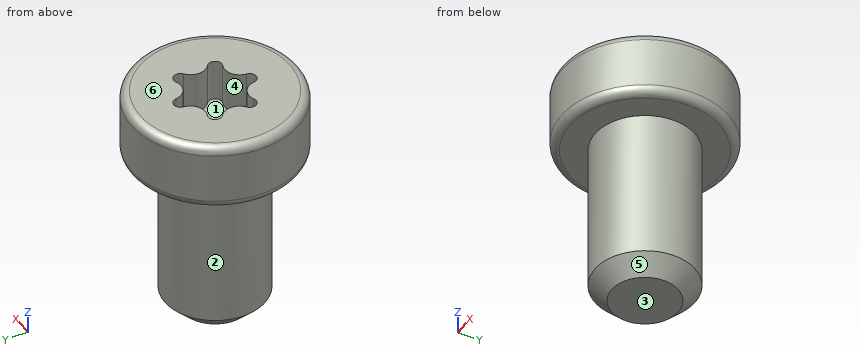
Solid Edge part; units mm, degrees
sketch "Sketch1" plane through (0, 0, 0) normal (0, -1, 0) x (1, 0, 0)
  line L0 (0, 4) -> (5, 4)
  line L1 (5, 4) -> (5, 0)
  line L2 (5, 0) -> (3, 0)
  line L3 (3, 0) -> (3, -10)
  line L4 (3, -10) -> (0, -10)
  line L5 (0, -10) -> (0, 4)
  dimension "D1" = 3
  dimension "D2" = 3
  dimension "D3" = 5
revolve "RevolvedProtrusion1" add sketch "Sketch1" angle 360 about axis through (0, 0, 54) along (0, 0, -1)
sketch "Sketch2" plane through (0, 0, 4) normal (0, 0, 1) x (1, 0, 0)
  arc A0 (-2.0545, -0.7268) -> (-1.6567, -1.4158) centre (-1.8186, -1.05) ccw
  arc A1 (-1.6567, -1.4158) -> (-0.3978, -2.1427) centre (-1.2926, -2.2389) cw
  arc A2 (-0.3978, -2.1427) -> (0.3978, -2.1427) centre (0, -2.0999) ccw
  arc A3 (0.3978, -2.1427) -> (1.6567, -1.4158) centre (1.2926, -2.2389) cw
  arc A4 (1.6567, -1.4158) -> (2.0545, -0.7268) centre (1.8186, -1.05) ccw
  arc A5 (2.0545, -0.7268) -> (2.0545, 0.7268) centre (2.5853, 0) cw
  arc A6 (2.0545, 0.7268) -> (1.6567, 1.4158) centre (1.8186, 1.05) ccw
  arc A7 (1.6567, 1.4158) -> (0.3978, 2.1427) centre (1.2926, 2.2389) cw
  arc A8 (0.3978, 2.1427) -> (-0.3978, 2.1427) centre (0, 2.0999) ccw
  arc A9 (-0.3978, 2.1427) -> (-1.6567, 1.4158) centre (-1.2926, 2.2389) cw
  arc A10 (-1.6567, 1.4158) -> (-2.0545, 0.7268) centre (-1.8186, 1.05) ccw
  arc A11 (-2.0545, 0.7268) -> (-2.0545, -0.7268) centre (-2.5853, 0) cw
extrude "Cutout1" cut sketch "Sketch2" against normal blind 2.5
fillet "Verrundung_1" radius 0.5 2 edges at (-5, 0, 4) (-5, 0, 0)
chamfer "Fase_1" distance 1 angle 45 1 edges at (-3, 0, -10)
The listing builds one solid part. Answer for the finished solid, in the listing's coordinates (mm). Face numbers are marked on the shaded views. A direction names the side the tool comes from. Give positions to 0.01 mm unless a question says otherwise; leave off trailing zeros. Order: outer loops, then holes, each group sorted by start corner. A loop starts at its lowest first (then second) coordinate and runs counter-clockwise, first axis right, second up. Notation, with made-up numbers: M 5.25,12.25 L 12.25,12.25 A22 cw 12.25,25.25 Z; hole C 68,2 d10. An arc over 180 degrees is marked long. Put each result on its own line as item: value. Start each with the question number.
Item 1: For a pull along X with two mould halves and no side action, classify the marked faces 4, 5 and 6 as +X half, -X half, draft (parallel to the pull), parting line (faces both ways), or undercut.
Item 2: The part is cut by section C-C, the plane z = -4.5. Determine the outline of the cut face in (x, y).
Item 3: Flat-ended cylindrical pins translate along their axes: P1, Ø5, axis at x = -3.5, z = -4, coming from the +Y side; P2, Ø6, axis at x = 3, z = -2.5, coming from the -Y side; P3, Ø4, axis at x = 3, z = -3.5, coming from the -Y side. Find the tip coordinate at first contact, or state that the pin passes through.
Item 4: Which of the six approach directions +Z, -Z, +X, -X, +Y, -Y give full straight-line access (tool end or side, diameter ignored) to the marked faces 1, 2 and 3?
Item 5: Find the intervals of material crossed by line 1 along Z through (x, y) = (0.75, 0.25); line 2 along X through (y, z) = (-0.5, 3); line 3 along Z through (x, y) = (3.5, 2), in increasing order.
Item 6: The part is cut by section A-A, the plane y = 0. Determine the outline of the cut face in (x, z), and give its area (3 significant figures).
Item 7: The part is cut by section B-B, the plane x = 0. Determine the outline of the cut face in (y, z), and give its area (3 significant figures).
Answer key:
1. face 4: undercut
1. face 5: parting line
1. face 6: draft
2. outline: C 0,0 d6
3. P1: stops at y = 2.83
3. P2: stops at y = -4.6
3. P3: stops at y = -2.83
4. face 1: +Z
4. face 2: -Z
4. face 3: -Z, +X, -X, +Y, -Y
5. line 1: z = -10 to 1.5
5. line 2: x = -4.97 to -1.84, 1.84 to 4.97
5. line 3: z = 0 to 4
6. outline: M -5,0.5 A0.5 ccw -4.5,0 L -3,0 L -3,-9 L -2,-10 L 2,-10 L 3,-9 L 3,0 L 4.5,0 A0.5 ccw 5,0.5 L 5,3.5 A0.5 ccw 4.5,4 L 1.69,4 L 1.69,1.5 L -1.69,1.5 L -1.69,4 L -4.5,4 A0.5 ccw -5,3.5 Z
6. area: 90.4 mm²
7. outline: M -5,0.5 A0.5 ccw -4.5,0 L -3,0 L -3,-9 L -2,-10 L 2,-10 L 3,-9 L 3,0 L 4.5,0 A0.5 ccw 5,0.5 L 5,3.5 A0.5 ccw 4.5,4 L 2.5,4 L 2.5,1.5 L -2.5,1.5 L -2.5,4 L -4.5,4 A0.5 ccw -5,3.5 Z
7. area: 86.3 mm²
